Can you work these out from the model? Positions are in its coordinate system, mm. Give positions to 0.01 mm unless a question says otherwise; leave off trailing zeros. Write each loop counter-clockwise with the first axis right and the second up, starting at its lowest first coordinate (ties: lowest second). Pieces come first, ordered by that corner, then holes. Notation, with made-up numbers: M 44.5,-3 L 52.5,-3 A38 ccw 52.5,35 Z; hole C 74.5,-9 d4. An arc over 180 degrees is marked long. Use CSV: the item, a comma, the result in double quotes. Start each with the question number.
from build123d import *

# Parameters (mm, degrees)
ESBO_O2_R                = 32.5
RESSALTO_EXTRUS_O1_DEPTH = 40
ESBO_O3_R                = 28.5
CORTE_EXTRUS_O1_DEPTH    = 40
ESBO_O4_W                = 30
ESBO_O4_H                = 19.489170569
CORTE_EXTRUS_O2_DEPTH    = 61.930288035


with BuildPart() as part:
    # Esboço2 → Ressalto-extrusão1 (new body)
    with BuildSketch(Plane(origin=(0, 0, 0), x_dir=(1, 0, 0), z_dir=(0, 1, 0))):
        with Locations(Location((0, 0, 0), (0, 0, 270))):
            Circle(ESBO_O2_R)
    extrude(amount=RESSALTO_EXTRUS_O1_DEPTH)

    # Esboço3 → Corte-extrusão1 (cut)
    with BuildSketch(Plane(origin=(0, 40, 0), x_dir=(1, 0, 0), z_dir=(0, 1, 0))):
        with Locations(Location((0, 0, 0), (0, 0, 270))):
            Circle(ESBO_O3_R)
    extrude(amount=-CORTE_EXTRUS_O1_DEPTH, mode=Mode.SUBTRACT)

    # Esboço4 → Corte-extrusão2 (cut, through all)
    with BuildSketch(Plane(origin=(0, 0, 0), x_dir=(1, 0, 0), z_dir=(0, 1, 0))):
        with Locations((0, -26.797609532)):
            Rectangle(ESBO_O4_W, ESBO_O4_H)
    extrude(amount=CORTE_EXTRUS_O2_DEPTH, mode=Mode.SUBTRACT)


solid = part.part
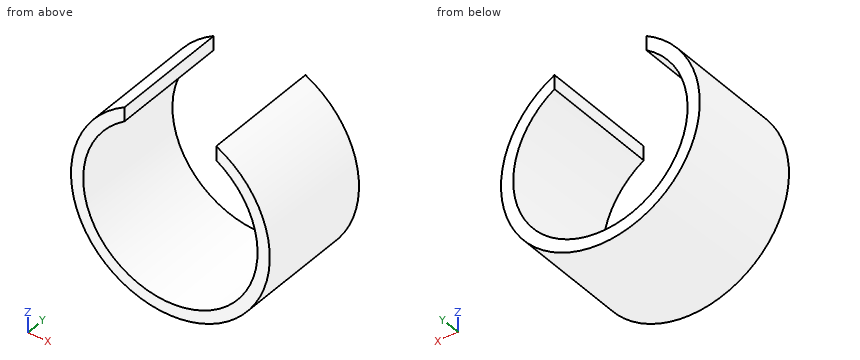
(1) I want a section at A-A (z = 0). Write out the boundary of the cut face in (x, y), and give its area (3 significant figures).
(2) I want a section at B-B (x = 18). Write out the boundary of the cut face in (y, z).
(3) I want a section at D-D (x = 0). Write out the boundary of the cut face in (y, z), and give its area (3 significant figures).
(4) Will these pins go through, and if not, where does the flat tip stop? pin 1 Ø1.5 at (x, y) = (25.5, 26.5) entering from +Z; pin 2 Ø1.4 at (y, z) = (11, 26.5) entering from -X; pin 3 Ø5 at (y, z) = (27.5, 5.5) entering from -X; pin 4 Ø8 at (x, z) = (23, 1.5) entering from -Y.
(5) I want a section at C-C (y = 9.5). Write out the boundary of the cut face in (x, z).
(6) Please list where these lines run through material, in increasing order: L1, parallel to X at y = 31, z = 0; L2, parallel to Z at x = 0, y = 17; L3, parallel to X at y = 13.5, z = -14.5. Write a range as [from, to].
Geometry results:
1,outline,"M -32.5,0 L -28.5,0 L -28.5,40 L -32.5,40 Z; M 28.5,0 L 32.5,0 L 32.5,40 L 28.5,40 Z"
1,area,"320 mm2"
2,outline,"M 0,-27.06 L 40,-27.06 L 40,-22.1 L 0,-22.1 Z; M 0,22.1 L 40,22.1 L 40,27.06 L 0,27.06 Z"
3,outline,"M 0,-32.5 L 40,-32.5 L 40,-28.5 L 0,-28.5 Z"
3,area,"160 mm2"
4,pin 1,"stops at z = 21.06"
4,pin 2,"stops at x = -19.76"
4,pin 3,"stops at x = -32.36"
4,pin 4,"passes through"
5,outline,"M -15,24.23 L -15,28.83 A32.5 ccw long 15,28.83 L 15,24.23 A28.5 cw long Z"
6,L1,"x = [-32.5, -28.5], [28.5, 32.5]"
6,L2,"z = [-32.5, -28.5]"
6,L3,"x = [-29.09, -24.54], [24.54, 29.09]"
